Drawing for the job (mm, zero at the part's lowest x, y, z). A direction names the side the tool comes from. Coordinates: 2 decimals unless noted, no trailing zeros. Write each loop counter-clockwise with the first axis right and the second up, starting at its lowest first coordinate (ties: lowest second). Pieces come first, ordered by that corner, then holes. Notation, with made-up numbers: M 27.5,-31 L 59.5,-31 A23 cw 59.5,-6 Z; hole C -21.5,-10 d7. An arc over 180 degrees is marked long. Put each result on its own line as item: value. Start each with the question number.
Q1. Cut at C-C (y = 39). Write the cut outline in (x, z), then the cut area to 3 significant figures.
Q2. Drop flat-ended pins along their axis: pin 1 (4 mm diameter, centred on y = 39, z = 59.5, fed in from +X); pin 2 (2.5 mm diameter, centred on y = 53.5, z = 49, fed in from +X); pin 3 (4 mm diameter, centred on x = 84.5, z = 35.5, fed in from +Y). Give the stop position or say it passes through.
Q3. Cut at B-B (x = 32). Write the cut outline in (y, z), then the cut area to 3 significant figures.
Q4. Pull direction X, two halves, no side cores. Call the marked faces 4, 5 and 6: pulls with the +X half, pulls with the -X half, needs draft (parallel to the pull), parting line crosses it, or undercut.
Q5. Cut at A-A (z = 25). Write the cut outline in (x, y).
Q6. Which spindle directions (+Z, -Z, +X, -X, +Y, -Y) get a long thin tool onto all of the face, cutting with end or side? Do the marked faces 1, 2 and 3. Say none if no direction does.
Q7. Drill centre lines: line 1 along X through (y, z) = (30.5, 34.5); line 2 along X through (y, z) = (53, 23); line 3 along Y through (x, z) = (54.5, 23.5). Where is each one in solid material? Low to high.
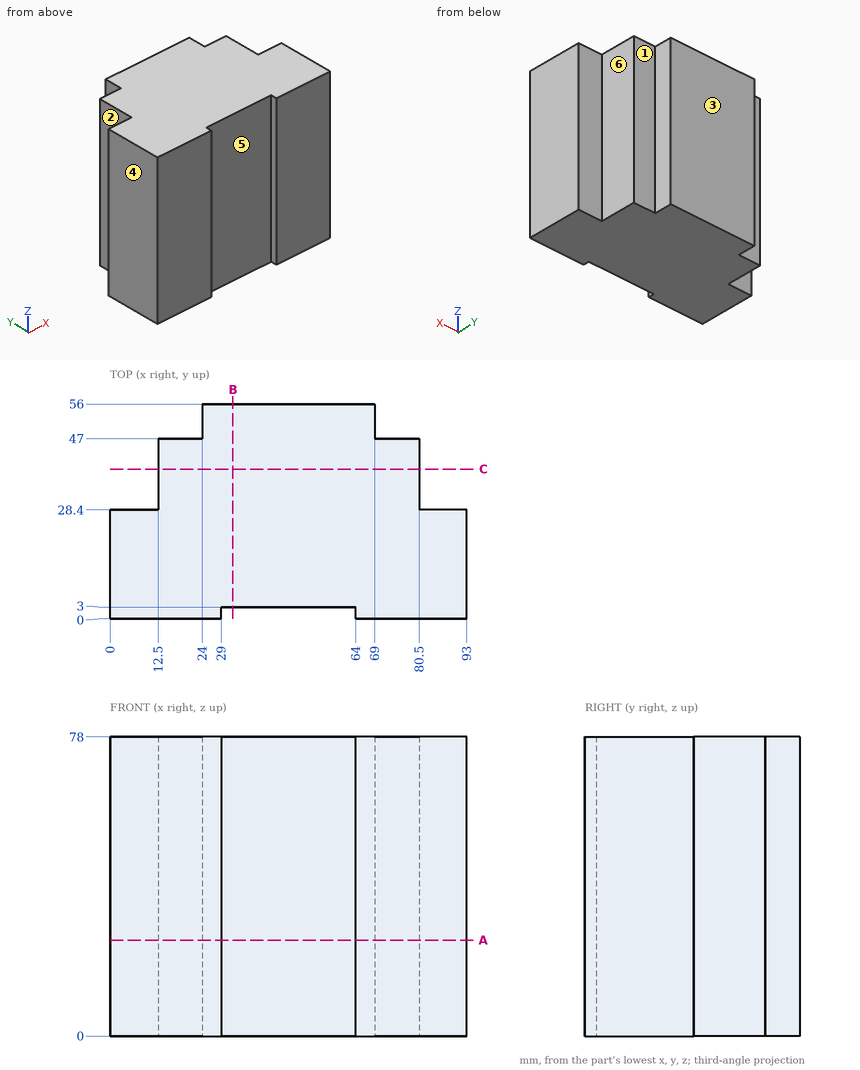
Computed values:
1. outline: M 12.5,0 L 80.5,0 L 80.5,78 L 12.5,78 Z
1. area: 5,300 mm2
2. pin 1: x = 80.5
2. pin 2: x = 69
2. pin 3: y = 28.4
3. outline: M 3,0 L 56,0 L 56,78 L 3,78 Z
3. area: 4,130 mm2
4. face 4: pulls with the -X half
4. face 5: undercut
4. face 6: pulls with the +X half
5. outline: M 0,0 L 29,0 L 29,3 L 64,3 L 64,0 L 93,0 L 93,28.4 L 80.5,28.4 L 80.5,47 L 69,47 L 69,56 L 24,56 L 24,47 L 12.5,47 L 12.5,28.4 L 0,28.4 Z
6. face 1: +Z, -Z, +X, +Y
6. face 2: +Z, -Z, -X, +Y
6. face 3: +Z, -Z, +X, -X, +Y
7. line 1: 12.5 to 80.5
7. line 2: 24 to 69
7. line 3: 3 to 56
